from build123d import *

# Parameters (mm, degrees)
BOSS_EXTRUDE3_OUTLINE_R = 3
BOSS_EXTRUDE3_DEPTH     = 98
SKETCH3_R               = 3
BOSS_EXTRUDE4_DEPTH     = 5
CUT_EXTRUDE6_DEPTH      = 144.320079016
CUT_EXTRUDE6_DEPTH_BACK = 144.320079016
CUT_EXTRUDE9_DEPTH      = 98
SKETCH10_W              = 0.4
SKETCH10_H              = 1.8
SKETCH10_W_2            = 1.8
SKETCH10_H_2            = 0.4
SKETCH10_H_3            = 1.6
SKETCH10_W_3            = 1.6
BOSS_EXTRUDE5_DEPTH     = 98
SKETCH11_W              = 75
SKETCH11_H              = 43.392810524
CUT_EXTRUDE10_DEPTH     = 10


# Read off the part's stored shape, not the designer's step: Boss-Extrude3
with BuildPart() as part:
    # Boss-Extrude3 outline → Boss-Extrude3 (new body)
    with BuildSketch(Plane.XY):
        with BuildLine():
            ThreePointArc((-24.392810524, 72.348554199), (-55.939709188, 51.962211615), (-73.948106805, 19))
            Line((-73.948106805, 19), (-53.527635725, 19))
            add(Edge.make_bspline(
                [(-72.348554199, -24.392810524), (-69.541086329, -27.040667073), (-67.428574969, -29.089162938), (-64.355831171, -30.241441862), (-60.963009895, -31.073643307), (-59.042545022, -30.561519341), (-56.673971678, -29.217193929), (-54.241382838, -27.488775543), (-53, -25.105954954), (-53, -17.37432721), (-53.527635725, 19)],
                knots=[0, 0, 0, 0, 0, 0, 0, 0, 0, 0, 0, 1, 1, 1, 1, 1, 1, 1, 1, 1, 1, 1], degree=10))
            ThreePointArc((-72.348554199, -24.392810524), (-51.962211615, -55.939709188), (-19, -73.948106805))
            Line((-19, -73.948106805), (-19, -53))
            add(Edge.make_bspline(
                [(24.392810524, -72.348554199), (27.040667073, -69.541086329), (29.089162938, -67.428574969), (30.241441862, -64.355831171), (31.073643307, -60.963009895), (30.561519341, -59.042545022), (29.217193929, -56.673971678), (27.488775543, -54.241382838), (25.105954954, -53), (17.37432721, -53), (-19, -53)],
                knots=[0, 0, 0, 0, 0, 0, 0, 0, 0, 0, 0, 1, 1, 1, 1, 1, 1, 1, 1, 1, 1, 1], degree=10))
            ThreePointArc((24.392810524, -72.348554199), (55.939709188, -51.962211615), (73.948106805, -19))
            Line((73.948106805, -19), (52.782560411, -19))
            add(Edge.make_bspline(
                [(72.348554199, 24.392810524), (69.541086329, 27.040667073), (67.428574969, 29.089162938), (64.355831171, 30.241441862), (60.963009895, 31.073643307), (59.042545022, 30.561519341), (56.673971678, 29.217193929), (54.241382838, 27.488775543), (53, 25.105954954), (53, 17.37432721), (52.782560411, -19)],
                knots=[0, 0, 0, 0, 0, 0, 0, 0, 0, 0, 0, 1, 1, 1, 1, 1, 1, 1, 1, 1, 1, 1], degree=10))
            ThreePointArc((72.348554199, 24.392810524), (51.962211615, 55.939709188), (19, 73.948106805))
            Line((19, 73.948106805), (19, 53))
            add(Edge.make_bspline(
                [(-24.392810524, 72.348554199), (-27.040667073, 69.541086329), (-29.089162938, 67.428574969), (-30.241441862, 64.355831171), (-31.073643307, 60.963009895), (-30.561519341, 59.042545022), (-29.217193929, 56.673971678), (-27.488775543, 54.241382838), (-25.105954954, 53), (-17.37432721, 53), (19, 53)],
                knots=[0, 0, 0, 0, 0, 0, 0, 0, 0, 0, 0, 1, 1, 1, 1, 1, 1, 1, 1, 1, 1, 1], degree=10))
        make_face()
        with Locations((-30, -59)):
            Circle(BOSS_EXTRUDE3_OUTLINE_R, mode=Mode.SUBTRACT)
        with Locations((58.782560411, -30)):
            Circle(BOSS_EXTRUDE3_OUTLINE_R, mode=Mode.SUBTRACT)
        with Locations((-59.527635725, 30)):
            Circle(BOSS_EXTRUDE3_OUTLINE_R, mode=Mode.SUBTRACT)
        Polygon((-38.9, -51.6), (-51.6, -51.6), (-51.6, -38.9), (-50, -38.9), (-50, 38.9), (-51.6, 38.9), (-51.6, 51.6), (-38.9, 51.6), (-38.9, 50), (38.9, 50), (38.9, 51.6), (51.6, 51.6), (51.6, 38.9), (50, 38.9), (50, -38.9), (51.6, -38.9), (51.6, -51.6), (38.9, -51.6), (38.9, -50), (-38.9, -50), align=None, mode=Mode.SUBTRACT)
        with Locations((30, 59)):
            Circle(BOSS_EXTRUDE3_OUTLINE_R, mode=Mode.SUBTRACT)
    extrude(amount=BOSS_EXTRUDE3_DEPTH)

    # Sketch3 → Boss-Extrude4 (add)
    with BuildSketch(Plane.XY.offset(98)):
        with Locations((-59.527635725, 30)):
            Circle(SKETCH3_R)
    extrude(amount=BOSS_EXTRUDE4_DEPTH)


with BuildPart() as boss_extrude4_kept_piece:
    # of the separate pieces the step leaves, the one the design keeps (boss_extrude4_pieces_kept)
    add(part.part.solids().sort_by_distance((-24.392810524, 72.348554199, 0))[0])

    # Sketch5 → Cut-Extrude6 (cut, two sides: drawn at the far end of the back side and taken through both)
    with BuildSketch(Plane.XY.offset(98).offset(-CUT_EXTRUDE6_DEPTH_BACK)):
        Polygon((38.7, 51.8), (51.8, 51.8), (51.8, 38.7), (50.2, 38.7), (50.2, -38.7), (51.8, -38.7), (51.8, -51.8), (38.7, -51.8), (38.7, -50.2), (-38.7, -50.2), (-38.7, -51.8), (-51.8, -51.8), (-51.8, -38.7), (-50.2, -38.7), (-50.2, 38.7), (-51.8, 38.7), (-51.8, 51.8), (-38.7, 51.8), (-38.7, 50.2), (38.7, 50.2), align=None)
        Polygon((-38.9, -51.6), (-51.6, -51.6), (-51.6, -38.9), (-50, -38.9), (-50, 38.9), (-51.6, 38.9), (-51.6, 51.6), (-38.9, 51.6), (-38.9, 50), (38.9, 50), (38.9, 51.6), (51.6, 51.6), (51.6, 38.9), (50, 38.9), (50, -38.9), (51.6, -38.9), (51.6, -51.6), (38.9, -51.6), (38.9, -50), (-38.9, -50), align=None, mode=Mode.SUBTRACT)
    extrude(amount=CUT_EXTRUDE6_DEPTH + CUT_EXTRUDE6_DEPTH_BACK, mode=Mode.SUBTRACT)

    # Sketch6 → Cut-Extrude9 (cut)
    with BuildSketch(Plane.XY.offset(98)):
        Polygon((-51.8, 38.7), (-51.8, 51.8), (-38.7, 51.8), (-38.7, 52), (-52, 52), (-52, 38.7), align=None)
        Polygon((-38.7, -51.8), (-51.8, -51.8), (-51.8, -38.7), (-52, -38.7), (-52, -52), (-38.7, -52), align=None)
        Polygon((51.8, -38.7), (51.8, -51.8), (38.7, -51.8), (38.7, -52), (52, -52), (52, -38.7), align=None)
        Polygon((51.8, 38.7), (51.8, 51.8), (38.7, 51.8), (38.7, 51.6), (51.6, 51.6), (51.6, 38.7), align=None)
    extrude(amount=-CUT_EXTRUDE9_DEPTH, mode=Mode.SUBTRACT)

    # Sketch10 → Boss-Extrude5 (add)
    with BuildSketch(Plane.XY.offset(98)):
        with Locations((-38.9, 51.1)):
            Rectangle(SKETCH10_W, SKETCH10_H)
        with Locations((-51.1, 38.9)):
            Rectangle(SKETCH10_W_2, SKETCH10_H_2)
        with Locations((38.9, 51)):
            Rectangle(SKETCH10_W, SKETCH10_H_3)
        with Locations((51, 38.9)):
            Rectangle(SKETCH10_W_3, SKETCH10_H_2)
        with Locations((51.1, -38.9)):
            Rectangle(SKETCH10_W_2, SKETCH10_H_2)
        with Locations((38.9, -51.1)):
            Rectangle(SKETCH10_W, SKETCH10_H)
        with Locations((-51.1, -38.9)):
            Rectangle(SKETCH10_W_2, SKETCH10_H_2)
        with Locations((-38.9, -51.1)):
            Rectangle(SKETCH10_W, SKETCH10_H)
    extrude(amount=-BOSS_EXTRUDE5_DEPTH)

    # Sketch11 → Cut-Extrude10 (cut)
    with BuildSketch(Plane.ZY.offset(-50.2)):
        with Locations((49, 2.696405262)):
            Rectangle(SKETCH11_W, SKETCH11_H)
    extrude(amount=-CUT_EXTRUDE10_DEPTH, mode=Mode.SUBTRACT)


solid = boss_extrude4_kept_piece.part
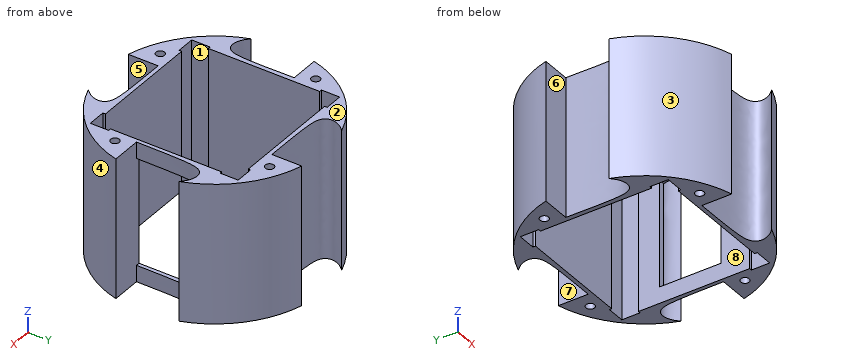
CAD build for the part. Positions are in the model's coordinates, mm. Face numbers are marked on the shaded views. A direction names the side the tool comes from. Round coordinates to 2 decimals unless told otherwise and drop trailing zeros. Loops run counter-clockwise (first coordinate to the right, second up) from the corner with the lowest first, then second, coordinate; pieces in that order, holes last.
(1) Wall check: line 1 along Y through (x, z) = (-0.5, 14); line 2 along Y through (x, z) = (-30, 57); line 3 along X through (y, z) = (25.5, 9.5). Give the ranges that are in metal, low to high.
(2) Cut at A-A (x = -35.5). Give the cut face in (y, z), plus the area to 3 significant figures.
(3) Two-plate mould, pull along X, no slides. Class the marked faces 1, 2 and 3: +X half, -X half, draft (parallel to the pull), parting line (faces both ways), or undercut.
(4) Cut at B-B (z = 69). State how many separate pieces and enclosed holes the cut face has, plus the area to 3 significant figures.
(5) Drop flat-ended pins along their axis: pin 1 (10.5 mm diameter, centred on x = -46, z = 43.5, fed in from -Y); pin 2 (6 mm diameter, centred on y = 56, z = 82.5, fed in from +X); pin 3 (4 mm diameter, centred on y = 44.5, z = 49.5, fed in from -X). Give the stop position or say it passes through.
(6) Which spindle directions (+Z, -Z, +X, -X, +Y, -Y) get a long thin tool onto all of the face, cutting with end or side? Do the marked faces 4, 5, 6, 7 and 8. Say none if no direction does.
Findings below:
1. line 1: y = -53.03 to -50.2, 50.2 to 53.04
1. line 2: y = -70.21 to -62, -56 to -50.2, 50.2 to 70.21
1. line 3: x = -71.97 to -50.2, 50.2 to 55.22, 71.16 to 71.97
2. outline: (-67.59, 0) - (-50.2, 0) - (-50.2, 98) - (-67.59, 98) - close; (50.2, 0) - (67.59, 0) - (67.59, 98) - (50.2, 98) - close
2. area: 3,410 mm2
3. face 1: undercut
3. face 2: draft
3. face 3: -X half
4. separate pieces: 1
4. enclosed holes: 4
4. area: 3,740 mm2
5. pin 1: stops at y = -64.57
5. pin 2: stops at x = 54.96
5. pin 3: stops at x = -63.43
6. face 4: +Z, -Z, +X, -Y
6. face 5: +Z, -Z, -Y
6. face 6: +Z, -Z, -X
6. face 7: +Z, -Z, +Y
6. face 8: +Z, -Z
